from build123d import *

# Parameters (mm, degrees)
F2_R      = 12.49045
F3_DEPTH  = 25.4
F5_W      = 16.0147
F5_H      = 15.9385
F6_DEPTH  = 12.0142
F7_R      = 2.8829
F7_R_2    = 0.9779
F8_DEPTH  = 25.4
F9_DEPTH  = 5.8166
F11_R     = 1.44145
F12_DEPTH = 25.4


with BuildPart() as f1:
    # F0 (on Front) → F1 (revolve)
    with BuildSketch(Plane.XZ):
        Polygon((0, 49.9999), (0, 0), (4.64185, 0), (12.49045, 0), (12.49045, 1.1811), (6.43255, 1.1811), (6.43255, 3.3937222222), (12.49045, 3.3937222222), (12.49045, 4.5748222222), (6.43255, 4.5748222222), (6.43255, 6.7874444444), (12.49045, 6.7874444444), (12.49045, 7.9685444444), (6.43255, 7.9685444444), (6.43255, 10.1811666667), (12.49045, 10.1811666667), (12.49045, 11.3622666667), (6.43255, 11.3622666667), (6.43255, 13.5748888889), (12.49045, 13.5748888889), (12.49045, 14.7559888889), (4.40055, 14.7559888889), (4.40055, 16.9686111111), (12.49045, 16.9686111111), (12.49045, 18.1497111111), (4.40055, 18.1497111111), (4.40055, 20.3623333333), (12.49045, 20.3623333333), (12.49045, 21.5434333333), (4.40055, 21.5434333333), (4.40055, 23.7560555556), (12.49045, 23.7560555556), (12.49045, 24.9371555556), (4.40055, 24.9371555556), (4.40055, 27.1497777778), (12.49045, 27.1497777778), (12.49045, 28.3308777778), (4.40055, 28.3308777778), (4.40055, 30.5435), (12.49045, 30.5435), (12.49045, 31.7246), (4.40055, 31.7246), (4.40055, 33.8582), (7.96925, 33.8582), (7.96925, 35.3822), (4.40055, 35.3822), (4.40055, 37.6555), (7.96925, 37.6555), (7.96925, 40.6146), (5.98805, 40.6146), (5.98805, 46.355), (7.96925, 46.355), (7.96925, 49.9999), align=None)
        Polygon((4.64185, 0), (0, 0), (0, -6.858), (2.91465, -6.858), (2.91465, -3.8481), (4.64185, -3.8481), (5.46735, -3.0226), (5.46735, -0.8255), align=None)
    revolve(axis=Axis((0, 0, 24.99995), (0, 0, 1)))

    # F2 (on Top) → F3 (cut)
    with BuildSketch(Plane.XY):
        Circle(F2_R)
        Polygon((4.7348639914, -2.733675), (0, -5.46735), (-4.7348639914, -2.733675), (-4.7348639914, 2.733675), (0, 5.46735), (4.7348639914, 2.733675), align=None, mode=Mode.SUBTRACT)
    extrude(amount=-F3_DEPTH, mode=Mode.SUBTRACT)

    # F5 (on offset) → F6 (join)
    with BuildSketch(Plane(origin=(0, 0, -6.858), x_dir=(1, 0, 0), z_dir=(0, 0, -1))):
        with Locations((3.0226, 0)):
            Rectangle(F5_W, F5_H)
    extrude(amount=F6_DEPTH)

    # F7 (on face) → F8 (cut)
    with BuildSketch(Plane(origin=(0, 7.96925, 0), x_dir=(-1, 0, 0), z_dir=(0, 1, 0))):
        with Locations((-6.68655, -13.8938)):
            Circle(F7_R)
        with Locations((-9.07415, -8.8138)):
            Circle(F7_R_2)
    extrude(amount=-F8_DEPTH, mode=Mode.SUBTRACT)

    # F7 (on face) → F9 (cut)
    with BuildSketch(Plane(origin=(0, 7.96925, 0), x_dir=(-1, 0, 0), z_dir=(0, 1, 0))):
        with Locations((-1.32715, -10.2616)):
            Circle(F7_R_2)
    extrude(amount=-F9_DEPTH, mode=Mode.SUBTRACT)

    # F11 (on plane+point) → F12 (cut)
    with BuildSketch(Plane(origin=(0, 0, -13.8938), x_dir=(1, 0, 0), z_dir=(0, 0, -1))):
        with Locations((6.68655, 0)):
            Circle(F11_R)
    extrude(amount=F12_DEPTH, mode=Mode.SUBTRACT)


solid = f1.part
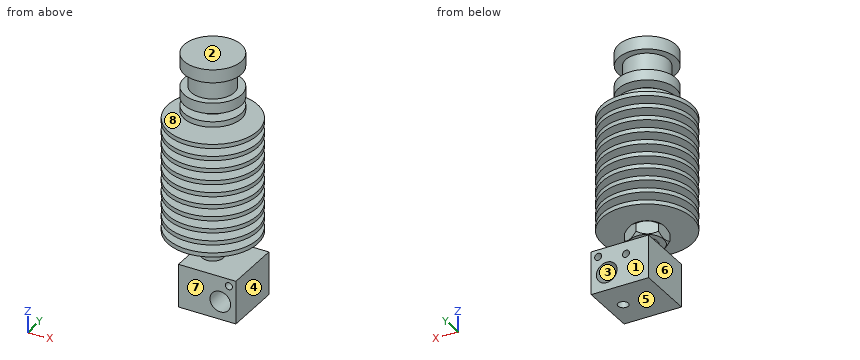
Check sheet for the modelled part. Datum: model origin and axes. Units: mm. Face numbers are marked on the shaded views. A direction names the side the tool comes from. Round coordinates to 2 decimals unless told otherwise and drop trailing zeros. Loops run counter-clockwise (first coordinate to the right, second up) from the corner with the lowest first, then second, coordinate; pieces in that order, holes last.
1. Sectioned sample at D-D on z = 44.5. Record the boundary of the cut face in (x, y), and give its area (3 significant figures).
2. Gauge pin test, flat ends, axial feed: pin 1 Ø4 at (y, z) = (-3.5, 21) entering from -X; pin 2 Ø8 at (x, z) = (-0.5, -8.5) entering from -Y; pin 3 Ø9 at (x, z) = (6.69, -13.89) entering from +Y. Record the tip position at first contact, or that the pin passes through.
3. Sectioned sample at B-B on y = 10.5. Give the number of separate pieces and of enclosed holes in the cut face, and give its area (3 significant figures).
4. Mould release check, pull along Z, two halves, no side actions. Record for the marked faces 1, 2 and 3: released by +Z, released by -Z, zero draft, split by the parting line, or undercut.
5. Sectioned sample at A-A on z = -4.5. Record the boundary of the cut face in (x, y), and give its area (3 significant figures).
6. Set-up check for the marked faces 4, 5, 6, 7 and 8: record each of +Z, -Z, +X, -X, +Y, -Y from which the full face is reachable in a straight line by a thin tool's end or side.
7. Scan lines: probe 1 along Y at (x, z) = (-2, -15); probe 2 along Y at (x, z) = (1.5, 19); probe 3 along X at (y, z) = (-2.25, 39). Record each from-to range of solid material in increasing order.
Recorded:
1. outline: circle Ø11.98 at (0, 0)
1. area: 113 mm2
2. pin 1: stops at x = -12.4
2. pin 2: stops at y = -7.97
2. pin 3: stops at y = 7.97
3. separate pieces: 10
3. enclosed holes: 0
3. area: 160 mm2
4. face 1: zero draft
4. face 2: released by +Z
4. face 3: undercut
5. outline: circle Ø5.83 at (0, 0)
5. area: 26.7 mm2
6. face 4: -Z, +X, +Y, -Y
6. face 5: -Z, +X, -X, +Y, -Y
6. face 6: -Z, -X, +Y, -Y
6. face 7: -Z, +X, -X, -Y
6. face 8: none
7. probe 1: y = -7.97 to 7.97
7. probe 2: y = -4.14 to 4.14
7. probe 3: x = -7.65 to 7.65
